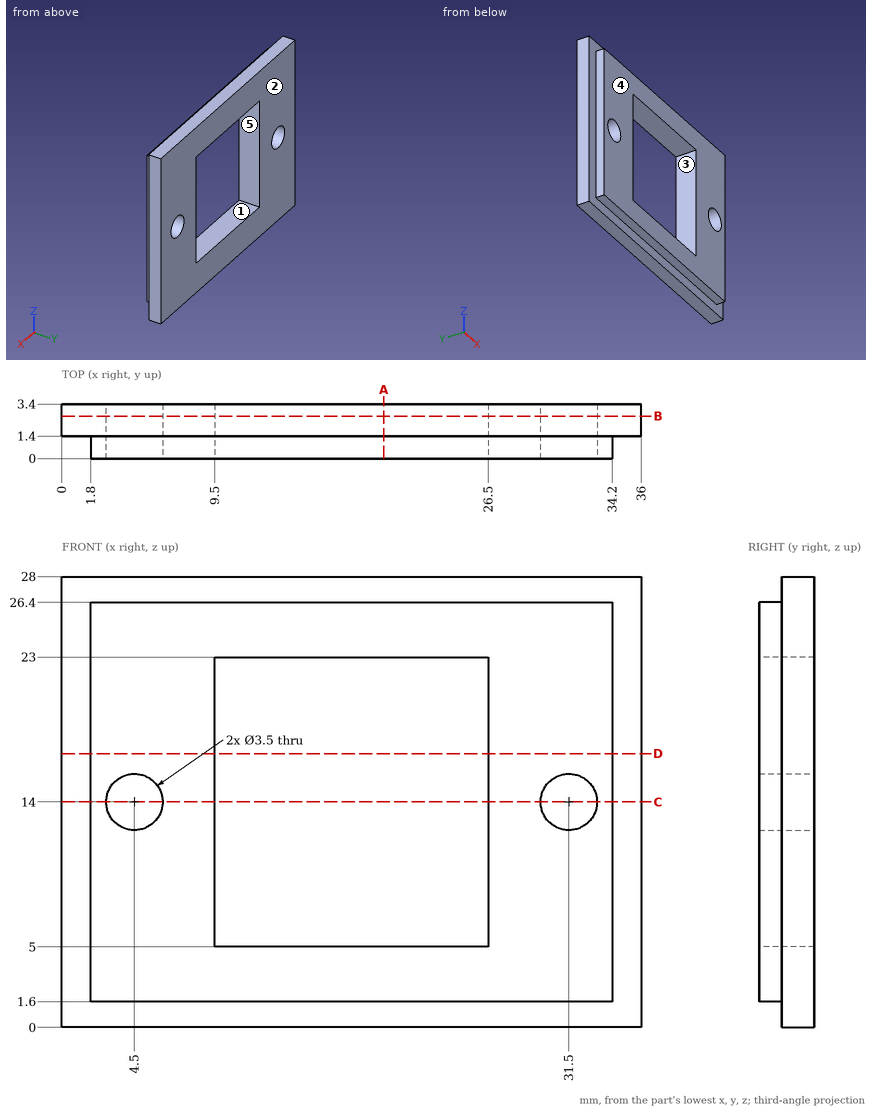
Geometry check sheet. Reference: drawing and pictorial views, mm from the part's lowest x, y, z. A direction names the side the tool comes from. Give positions to 0.01 mm unless a question says otherwise; leave off trailing zeros. Write each loop counter-clockwise with the first axis right and the second up, starting at its lowest first coordinate (ties: lowest second). Pieces come first, ordered by that corner, then holes. Notation, with made-up numbers: (18, 53) - (38, 53) arc R9 ccw to (38, 69) - close; hole circle Ø6 at (-19.5, 71.5). An arc over 180 degrees is marked (long way). Use a Markdown table: item, result.
Q1. Go/stop test with flat-tipped pins: P1, Ø0.7, axis at y = 0.5, z = 13, coming from the +X side; P2, Ø1.1, axis at y = 0.5, z = 19.5, coming from the -X side; P3, Ø1.1, axis at x = 18, y = 0.5, coming from the +Z side. Record where each tip stops, or that it passes through.
Computed:
| item | result |
|---|---|
| P1 | stops at x = 34.2 |
| P2 | stops at x = 1.8 |
| P3 | stops at z = 26.4 |
Q2. Draft check along Z on the marked faces 1, 2 and 3. Enter one of: pulls with the +Z half, pulls with the -Z half, needs draft (parallel to the pull), parting line crosses it, or undercut.
Computed:
| item | result |
|---|---|
| face 1 | undercut |
| face 2 | needs draft |
| face 3 | undercut |
Q3. Thickness scan on L1, parallel to X at y = 1.45, z = 14; L2, parallel to X at y = 1.25, z = 22.5; L3, parallel to Z at x = 31.5, y = 1.05. Record the ranges inside material, lowest first. Write a range as [from, to].
Computed:
| item | result |
|---|---|
| L1 | x = [0, 2.75], [6.25, 9.5], [26.5, 29.75], [33.25, 36] |
| L2 | x = [1.8, 9.5], [26.5, 34.2] |
| L3 | z = [1.6, 12.25], [15.75, 26.4] |
Q4. Set-up check for the marked faces 4 and 5: record each of +Z, -Z, +X, -X, +Y, -Y from which the full face is reachable in a straight line by a thin tool's end or side.
Computed:
| item | result |
|---|---|
| face 4 | +Z, -Z, +X, -X, -Y |
| face 5 | +Y, -Y |
Q5. Section check A-A, the plane x = 20. Enter the section's corners in (y, z).
Computed:
| item | result |
|---|---|
| outline | (0, 1.6) - (1.4, 1.6) - (1.4, 0) - (3.4, 0) - (3.4, 5) - (0, 5) - close; (0, 23) - (3.4, 23) - (3.4, 28) - (1.4, 28) - (1.4, 26.4) - (0, 26.4) - close |
Q6. Section check B-B, the plane y = 2.65. Enter the section's corners in (x, z).
Computed:
| item | result |
|---|---|
| outline | (0, 0) - (36, 0) - (36, 28) - (0, 28) - close; hole circle Ø3.5 at (4.5, 14); hole (9.5, 5) - (26.5, 5) - (26.5, 23) - (9.5, 23) - close; hole circle Ø3.5 at (31.5, 14) |
Q7. Section check C-C, the plane z = 14. Enter the section's corners in (x, y), then the cut area to 3 significant figures.
Computed:
| item | result |
|---|---|
| outline | (0, 1.4) - (1.8, 1.4) - (1.8, 0) - (2.75, 0) - (2.75, 3.4) - (0, 3.4) - close; (6.25, 0) - (9.5, 0) - (9.5, 3.4) - (6.25, 3.4) - close; (26.5, 0) - (29.75, 0) - (29.75, 3.4) - (26.5, 3.4) - close; (33.25, 0) - (34.2, 0) - (34.2, 1.4) - (36, 1.4) - (36, 3.4) - (33.25, 3.4) - close |
| area | 35.8 mm² |
Q8. Section check D-D, the plane z = 17. Enter the section's corners in (x, y), then the cut area to 3 significant figures.
Computed:
| item | result |
|---|---|
| outline | (0, 1.4) - (1.8, 1.4) - (1.8, 0) - (9.5, 0) - (9.5, 3.4) - (0, 3.4) - close; (26.5, 0) - (34.2, 0) - (34.2, 1.4) - (36, 1.4) - (36, 3.4) - (26.5, 3.4) - close |
| area | 59.6 mm² |
